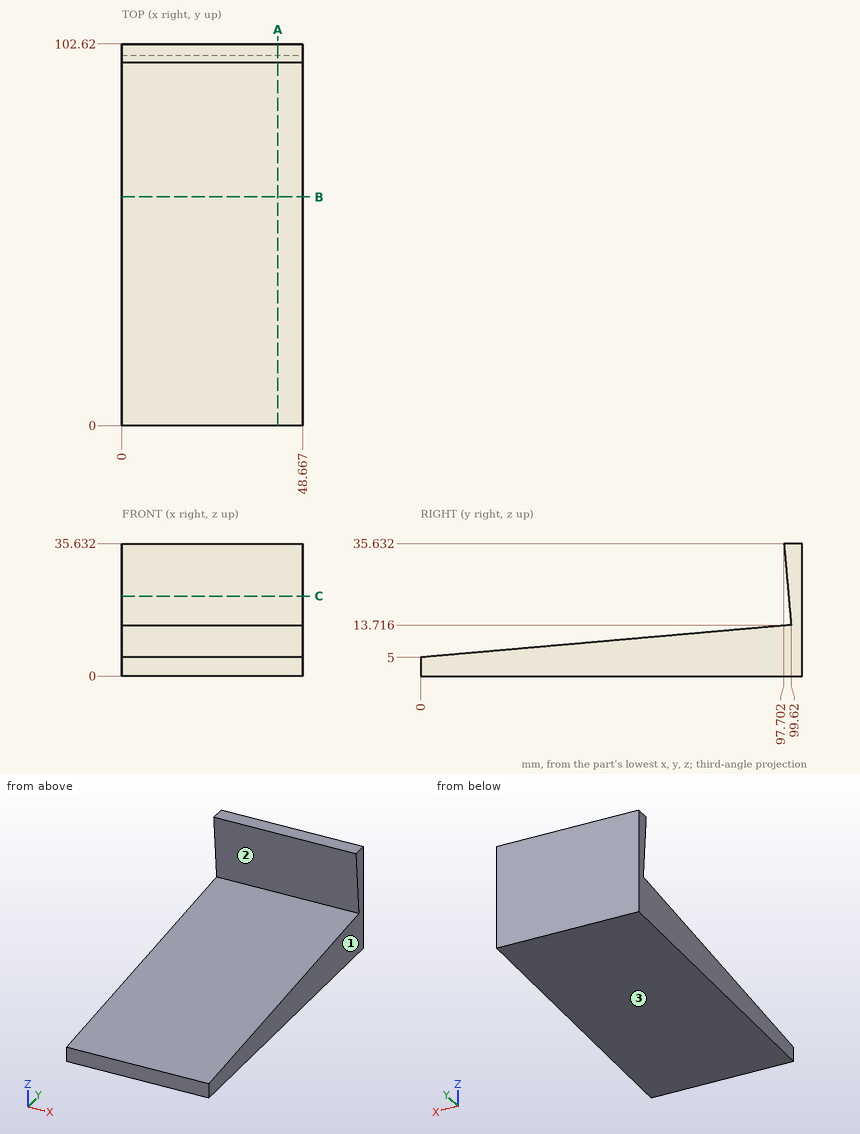
Source: three-view drawing plus pictorial views. Frame: mm from the lowest corner of the part. Round coordinates to 2 decimals unless told otherwise and drop trailing zeros. Loops run counter-clockwise (first coordinate to the right, second up) from the corner with the lowest first, then second, coordinate; pieces in that order, holes last. Notation, with made-up numbers: (-11, -26) - (4, -26) arc R18 cw to (4, -2) - close; hole circle Ø2 at (81.25, 80.25). An arc over 180 degrees is marked (long way). Write each question's results on one line, items separated by ' | '. Start each with the question number.
1) Cut plane B-B on y = 61.5. Return loops of the section in (x, z).
2) First-contact query: P1, Ø1, axis at x = 24, z = 15.5, coming from the -Y side; P2, Ø1.5, axis at y = 80, z = 13.5, coming from the -X side; P3, Ø1.5, axis at x = 39.5, y = 79.5, coming from the +Z side; P4, Ø8, axis at x = 44, y = 78.5, coming from the +Z side. Flat tips, straight axial feed; report the tip coordinate or a pass-through.
3) Mould query, pull axis Z, two halves, no side actions, for the marked faces 1, 2 and 3. Classes: released by +Z, released by -Z, zero draft, split by the parting line, or undercut.
4) Cut plane A-A on x = 42. Return loops of the section in (y, z) (1 decimal).
5) Cut plane C-C on z = 21.5. Return loops of the section in (x, y), then the cut area to 3 significant figures.
6) Line query: probe 1 along Y at (x, z) = (26, 14) (1 decimal); probe 2 along Z at (x, y) = (18, 89.5); probe 3 along Z at (x, y) = (5, 16). Output: solid intervals per line, ascending. Write a range as [from, to].
Verdict:
1) outline: (0, 0) - (48.67, 0) - (48.67, 10.38) - (0, 10.38) - close
2) P1: stops at y = 99.42 | P2: passes through | P3: stops at z = 12.02 | P4: stops at z = 12.22
3) face 1: zero draft | face 2: undercut | face 3: released by -Z
4) outline: (0, 0) - (102.6, 0) - (102.6, 35.6) - (97.7, 35.6) - (99.6, 13.7) - (0, 5) - close
5) outline: (0, 98.94) - (48.67, 98.94) - (48.67, 102.62) - (0, 102.62) - close | area: 179 mm2
6) probe 1: y = [99.6, 102.6] | probe 2: z = [0, 12.83] | probe 3: z = [0, 6.4]
